Input: part model. Units: mm. Frame: model coordinates. A direction names the side the tool comes from. Give positions to 0.01 mm unless a question says otherwise; leave off trailing zeros. Loops run counter-clockwise (first coordinate to the right, second up) from the corner with the lowest first, then second, coordinate; pieces in that order, holes last. Notation, with made-up numbers: M 87.5,35 L 109.5,35 A23 cw 109.5,46 Z; hole C 41.5,15.5 d4. An arc over 180 degrees is marked long. Use a Markdown table: item, result. Add a question column.
from build123d import *

# Parameters (mm, degrees)
SKETCH1_W           = 6.35
SKETCH1_H           = 28.575
SKETCH1_H_2         = 6.35
SKETCH1_W_2         = 28.575
BOSS_EXTRUDE1_DEPTH = 7.62
SKETCH2_R           = 1.213900036
CUT_EXTRUDE1_DEPTH  = 46.543269536


with BuildPart() as part:
    # Sketch1 → Boss-Extrude1 (new body)
    with BuildSketch(Plane(origin=(0, 0, 0), x_dir=(1, 0, 0), z_dir=(0, 1, 0))):
        with Locations((0, 17.4625)):
            Rectangle(SKETCH1_W, SKETCH1_H)
        Rectangle(SKETCH1_W, SKETCH1_H_2)
        with Locations((0, -17.4625)):
            Rectangle(SKETCH1_W, SKETCH1_H)
        with Locations((17.4625, 0)):
            Rectangle(SKETCH1_W_2, SKETCH1_H_2)
        with Locations((-17.4625, 0)):
            Rectangle(SKETCH1_W_2, SKETCH1_H_2)
    extrude(amount=BOSS_EXTRUDE1_DEPTH)

    # Sketch2 → Cut-Extrude1 (cut, through all)
    with BuildSketch(Plane(origin=(0, 7.62, 0), x_dir=(1, 0, 0), z_dir=(0, 1, 0))):
        with Locations(Location((0, 0, 0), (0, 0, 270))):
            Circle(SKETCH2_R)
    extrude(amount=-CUT_EXTRUDE1_DEPTH, mode=Mode.SUBTRACT)


solid = part.part
1) Section query D-D, the plane z = 25.5. Return the cut outline in (x, y) (3 decimals).
2) Section query B-B, the plane y = 3.25. Return the cut outline in (x, z) (3 decimals), and give its area (4 significant figures).
3) Section query A-A, the plane z = 0. Return the cut outline in (x, y), and give its area (3 significant figures).
4) Section query C-C, the plane x = 0. Return the cut outline in (y, z).
5) Reachability of faces 4 (the flat face through (-3.175, 4, -18)), 5 (the flat face through (3.175, 4, -17)), 6 (the flat face through (0, 7.62, -3)), 7 (the flat face through (-18, 4, 3.175)), 8 (the flat face through (3.175, 4, 18)) from +Z, -Z, +X, -X, +Y, -Y: full face, straight path, thin tool, end or side. Return the list, or none.
6) Ray query, line 1 (X direction, y = 2.5, z = 0); line 2 (Z direction, x = 29, y = 5.75) (3 decimals). Return the intervals inside material, ascending. Write a range as [from, to].
7) Pull-direction query (Z, two-part tool) for faces 1 (the flat face through (-3.175, 4, 17)), 2 (the cylindrical face through (-1.185, 3.863, -0.263)), 3 (the flat face through (0, 4, -31.75)); classes: pulls with the +Z half, pulls with the -Z half, needs draft (parallel to the pull), parting line crosses it, or undercut.
8) Contact query for flat-ended pins moving along their axis: P1, Ø4, axis at x = -3.5, z = 19.5, coming from the -Y side; P2, Ø4, axis at y = 3, z = -11.5, coming from the -X side (3 decimals); P3, Ø2, axis at x = -13, y = 2.5, coming from the -Z side (3 decimals); P4, Ø2, axis at x = -14.5, y = 2.5, coming from the +Z side (3 decimals). Output: stop coordinate, or through.
Entries:
| question | item | result |
|---|---|---|
| 1 | outline | M -3.175,0 L 3.175,0 L 3.175,7.62 L -3.175,7.62 Z |
| 2 | outline | M -31.75,-3.175 L -3.175,-3.175 L -3.175,-31.75 L 3.175,-31.75 L 3.175,-3.175 L 31.75,-3.175 L 31.75,3.175 L 3.175,3.175 L 3.175,31.75 L -3.175,31.75 L -3.175,3.175 L -31.75,3.175 Z; hole C 0,0 d2.428 |
| 2 | area | 761.5 mm² |
| 3 | outline | M -31.75,0 L -1.21,0 L -1.21,7.62 L -31.75,7.62 Z; M 1.21,0 L 31.75,0 L 31.75,7.62 L 1.21,7.62 Z |
| 3 | area | 465 mm² |
| 4 | outline | M 0,-31.75 L 7.62,-31.75 L 7.62,-1.21 L 0,-1.21 Z; M 0,1.21 L 7.62,1.21 L 7.62,31.75 L 0,31.75 Z |
| 5 | face 4 | -Z, -X, +Y, -Y |
| 5 | face 5 | -Z, +X, +Y, -Y |
| 5 | face 6 | +Z, -Z, +X, -X, +Y |
| 5 | face 7 | +Z, -X, +Y, -Y |
| 5 | face 8 | +Z, +X, +Y, -Y |
| 6 | line 1 | x = [-31.75, -1.21], [1.21, 31.75] |
| 6 | line 2 | z = [-3.175, 3.175] |
| 7 | face 1 | needs draft |
| 7 | face 2 | undercut |
| 7 | face 3 | pulls with the -Z half |
| 8 | P1 | stops at y = 0 |
| 8 | P2 | stops at x = -3.175 |
| 8 | P3 | stops at z = -3.175 |
| 8 | P4 | stops at z = 3.175 |
